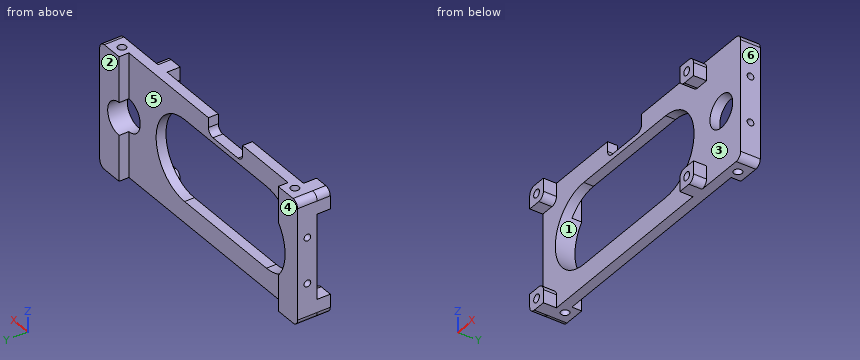
from build123d import *

# Parameters (mm, degrees)
BOSS_EXTRUDE1_DEPTH          = 38
FILLET3_R                    = 2
CUT_EXTRUDE1_DEPTH           = 98.349792201
CUT_EXTRUDE1_DEPTH_BACK      = 98.349792201
SKETCH3_W                    = 15
SKETCH3_H                    = 5
M3X0_5_TAPPED_HOLE3_D        = 2.5
M3X0_5_TAPPED_HOLE3_DEPTH    = 7.5
M3X0_5_TAPPED_HOLE3_TIP      = 0.751075774
M3X0_5_TAPPED_HOLE4_D        = 2.5
M3X0_5_TAPPED_HOLE4_DEPTH    = 7.5
M3X0_5_TAPPED_HOLE4_TIP      = 0.751075774
M2_5X0_45_TAPPED_HOLE1_D     = 2.05
M2_5X0_45_TAPPED_HOLE1_DEPTH = 6.35
M2_5X0_45_TAPPED_HOLE1_TIP   = 0.615882135
M2_5X0_45_TAPPED_HOLE2_D     = 2.05
M2_5X0_45_TAPPED_HOLE2_DEPTH = 6.35
M2_5X0_45_TAPPED_HOLE2_TIP   = 0.615882135
SKETCH14_R                   = 5
CUT_EXTRUDE2_DEPTH           = 98.488368751
SKETCH16_W                   = 6
SKETCH16_H                   = 6
BOSS_EXTRUDE2_DEPTH          = 4
FILLET4_R                    = 2
M3X0_5_TAPPED_HOLE5_D        = 2.5
M3X0_5_TAPPED_HOLE5_DEPTH    = 5.5
M3X0_5_TAPPED_HOLE5_TIP      = 0.751075774


with BuildPart() as part:
    # Sketch2 → Boss-Extrude1 (new body)
    with BuildSketch(Plane.XY.offset(11)):
        Polygon((-84.06534388, 85.95185693), (-75.56534388, 85.95185693), (-75.56534388, 82.95185693), (-5.56534388, 82.95185693), (-5.56534388, 85.95185693), (2.93465612, 85.95185693), (2.93465612, 79.95185693), (-84.06534388, 79.95185693), align=None)
    extrude(amount=BOSS_EXTRUDE1_DEPTH)

    # Fillet3
    fillet3_edges = [part.edges().sort_by_distance(p)[0] for p in [
        (2.93465612, 82.95185693, 49),
        (-84.06534388, 82.95185693, 11),
        (-84.06534388, 82.95185693, 49),
        (2.93465612, 82.95185693, 11),
    ]]
    fillet(fillet3_edges, radius=FILLET3_R)

    # Sketch3 → Cut-Extrude1 (cut, two sides: drawn at the far end of the back side and taken through both)
    with BuildSketch(Plane(origin=(0, 82.95185693, 0), x_dir=(1, 0, 0), z_dir=(0, 1, 0)).offset(-CUT_EXTRUDE1_DEPTH_BACK)):
        with BuildLine():
            Line((-66.06534388, -42.5), (-30.06534388, -42.5))
            ThreePointArc((-30.06534388, -42.5), (-17.56534388, -30), (-30.06534388, -17.5))
            Line((-30.06534388, -17.5), (-66.06534388, -17.5))
            ThreePointArc((-66.06534388, -17.5), (-78.56534388, -30), (-66.06534388, -42.5))
        make_face()
        with Locations((-48.06534388, -46.5)):
            Rectangle(SKETCH3_W, SKETCH3_H)
    extrude(amount=CUT_EXTRUDE1_DEPTH + CUT_EXTRUDE1_DEPTH_BACK, mode=Mode.SUBTRACT)

    # M3x0.5 Tapped Hole3
    with Locations(Plane.XY.offset(49)):
        with Locations((-78.56534388, 82.95185693), (-2.56534388, 82.95185693)):
            Hole(M3X0_5_TAPPED_HOLE3_D / 2, depth=M3X0_5_TAPPED_HOLE3_DEPTH)
            with Locations((0, 0, -(M3X0_5_TAPPED_HOLE3_DEPTH + M3X0_5_TAPPED_HOLE3_TIP / 2))):  # 118° drill point
                Cone(0, M3X0_5_TAPPED_HOLE3_D / 2, M3X0_5_TAPPED_HOLE3_TIP, mode=Mode.SUBTRACT)

    # M3x0.5 Tapped Hole4
    with Locations(Plane(origin=(0, 0, 11), x_dir=(-1, 0, 0), z_dir=(0, 0, -1))):
        with Locations((2.56534388, 82.95185693), (78.56534388, 82.95185693)):
            Hole(M3X0_5_TAPPED_HOLE4_D / 2, depth=M3X0_5_TAPPED_HOLE4_DEPTH)
            with Locations((0, 0, -(M3X0_5_TAPPED_HOLE4_DEPTH + M3X0_5_TAPPED_HOLE4_TIP / 2))):  # 118° drill point
                Cone(0, M3X0_5_TAPPED_HOLE4_D / 2, M3X0_5_TAPPED_HOLE4_TIP, mode=Mode.SUBTRACT)

    # M2.5x0.45 Tapped Hole1
    with Locations(Plane.ZY.offset(84.06534388)):
        with Locations((23, 82.95185693), (37, 82.95185693)):
            Hole(M2_5X0_45_TAPPED_HOLE1_D / 2, depth=M2_5X0_45_TAPPED_HOLE1_DEPTH)
            with Locations((0, 0, -(M2_5X0_45_TAPPED_HOLE1_DEPTH + M2_5X0_45_TAPPED_HOLE1_TIP / 2))):  # 118° drill point
                Cone(0, M2_5X0_45_TAPPED_HOLE1_D / 2, M2_5X0_45_TAPPED_HOLE1_TIP, mode=Mode.SUBTRACT)

    # M2.5x0.45 Tapped Hole2
    with Locations(Plane(origin=(2.93465612, 0, 0), x_dir=(0, 0, -1), z_dir=(1, 0, 0))):
        with Locations((-37, 82.95185693), (-23, 82.95185693)):
            Hole(M2_5X0_45_TAPPED_HOLE2_D / 2, depth=M2_5X0_45_TAPPED_HOLE2_DEPTH)
            with Locations((0, 0, -(M2_5X0_45_TAPPED_HOLE2_DEPTH + M2_5X0_45_TAPPED_HOLE2_TIP / 2))):  # 118° drill point
                Cone(0, M2_5X0_45_TAPPED_HOLE2_D / 2, M2_5X0_45_TAPPED_HOLE2_TIP, mode=Mode.SUBTRACT)

    # Sketch14 → Cut-Extrude2 (cut, through all)
    with BuildSketch(Plane(origin=(0, 85.95185693, 0), x_dir=(1, 0, 0), z_dir=(0, 1, 0))):
        with Locations(Location((-5.56534388, -30, 0), (0, 0, 270))):
            Circle(SKETCH14_R)
    extrude(amount=-CUT_EXTRUDE2_DEPTH, mode=Mode.SUBTRACT)

    # Sketch16 → Boss-Extrude2 (add)
    with BuildSketch(Plane.XZ.offset(-79.95185693)):
        with Locations((-81.06534388, 46)):
            Rectangle(SKETCH16_W, SKETCH16_H)
        with Locations((-81.06534388, 14)):
            Rectangle(SKETCH16_W, SKETCH16_H)
        with Locations((-15.06534388, 46)):
            Rectangle(SKETCH16_W, SKETCH16_H)
        with Locations((-15.06534388, 14)):
            Rectangle(SKETCH16_W, SKETCH16_H)
    extrude(amount=BOSS_EXTRUDE2_DEPTH)

    # Fillet4
    fillet4_edges = [part.edges().sort_by_distance(p)[0] for p in [
        (-12.06534388, 77.95185693, 11),
        (-84.06534388, 77.95185693, 11),
        (-84.06534388, 77.95185693, 49),
        (-78.06534388, 77.95185693, 43),
        (-78.06534388, 77.95185693, 17),
        (-18.06534388, 77.95185693, 17),
        (-18.06534388, 77.95185693, 43),
        (-12.06534388, 77.95185693, 49),
        (-40.56534388, 81.45185693, 44),
        (-55.56534388, 81.45185693, 44),
    ]]
    fillet(fillet4_edges, radius=FILLET4_R)

    # M3x0.5 Tapped Hole5
    with Locations(Plane.XZ.offset(-75.95185693)):
        with Locations((-81.06534388, 46), (-81.06534388, 14), (-15.06534388, 14), (-15.06534388, 46)):
            Hole(M3X0_5_TAPPED_HOLE5_D / 2, depth=M3X0_5_TAPPED_HOLE5_DEPTH)
            with Locations((0, 0, -(M3X0_5_TAPPED_HOLE5_DEPTH + M3X0_5_TAPPED_HOLE5_TIP / 2))):  # 118° drill point
                Cone(0, M3X0_5_TAPPED_HOLE5_D / 2, M3X0_5_TAPPED_HOLE5_TIP, mode=Mode.SUBTRACT)


solid = part.part
Geometry check sheet. Reference: the model listing, model coordinates, mm. Face numbers are marked on the shaded views. A direction names the side the tool comes from. Round coordinates to 2 decimals unless told otherwise and drop trailing zeros. Order: outer loops, then holes, each group sorted by start corner. A loop starts at its lowest first (then second) coordinate and runs counter-clockwise, first axis right, second up. Notation, with made-up numbers: (31.25, 41) -> (71.25, 41) arc R12 ccw to (71.25, 53) -> close; hole circle Ø5 at (-11, 74.5). An arc over 180 degrees is marked (long way). Use one line per item in the form item = value.
1. Cross-section at B-B, the plane y = 77. Enter the section's corners in (x, z), plus the area to 3 significant figures.
Working result:
outline = (-84.07, 13) arc R2 ccw to (-82.07, 11) -> (-78.07, 11) -> (-78.07, 15) arc R2 ccw to (-80.07, 17) -> (-84.07, 17) -> close; (-84.07, 43) -> (-80.07, 43) arc R2 ccw to (-78.07, 45) -> (-78.07, 49) -> (-82.07, 49) arc R2 ccw to (-84.07, 47) -> close; (-18.07, 11) -> (-14.07, 11) arc R2 ccw to (-12.07, 13) -> (-12.07, 17) -> (-16.07, 17) arc R2 ccw to (-18.07, 15) -> close; (-18.07, 45) arc R2 ccw to (-16.07, 43) -> (-12.07, 43) -> (-12.07, 47) arc R2 ccw to (-14.07, 49) -> (-18.07, 49) -> close; hole circle Ø2.5 at (-81.07, 14); hole circle Ø2.5 at (-81.07, 46); hole circle Ø2.5 at (-15.07, 14); hole circle Ø2.5 at (-15.07, 46)
area = 117 mm^2
2. Cross-section at C-C, the plane x = -63. Enter the section's corners in (y, z), plus the area to 3 significant figures.
Working result:
outline = (79.95, 11) -> (82.95, 11) -> (82.95, 17.5) -> (79.95, 17.5) -> close; (79.95, 42.5) -> (82.95, 42.5) -> (82.95, 49) -> (79.95, 49) -> close
area = 39.0 mm^2
3. Scan lines: line 1 along X through (y, z) = (82.75, 47); line 2 along X through (y, z) = (77.1, 46); line 3 along X through (y, z) = (85.75, 19.5). Record each from-to range of solid material in increasing order. Write a range as from..to.
Working result:
line_1 = -84.07..-79.8, -77.33..-55.57, -40.57..-3.8, -1.33..2.93
line_2 = -84.07..-82.32, -79.82..-78.07, -18.07..-16.32, -13.82..-12.07
line_3 = -84.07..-75.57, -5.57..2.93
4. Cross-section at D-D, the plane z = 32. Enter the section's corners in (x, y).
Working result:
outline = (-84.07, 79.95) -> (-78.4, 79.95) -> (-78.4, 85.95) -> (-84.07, 85.95) -> close; (-17.73, 79.95) -> (-10.15, 79.95) -> (-10.15, 82.95) -> (-17.73, 82.95) -> close; (-0.98, 79.95) -> (2.93, 79.95) -> (2.93, 85.95) -> (-0.98, 85.95) -> close
5. Go/stop test with flat-tipped pins: pin 1 (2 mm diameter, centred on x = -11, y = 78.5, fed in from -Z) (3 decimals); pin 2 (5 mm diameter, centred on x = -72.5, z = 16.5, fed in from +Y); pin 3 (3 mm diameter, centred on y = 78, z = 16, fed in from +X); pin 4 (2 mm diameter, centred on x = -2.57, y = 82.95, fed in from +Z). Record where each tip stops, or that it passes through.
Working result:
pin_1 = through
pin_2 = 82.95
pin_3 = -12.07
pin_4 = 41.35
6. Set-up check for the marked faces 1, 2 and 3: record each of +Z, -Z, +X, -X, +Y, -Y from which the full face is reachable in a straight line by a thin tool's end or side.
Working result:
face_1 = +Y, -Y
face_2 = +Z, -Z, +X, -X, +Y
face_3 = -Y
7. Cross-section at A-A, the plane y = 85. Enter the section's corners in (x, z), plus the area to 3 significant figures.
Working result:
outline = (-84.07, 13) arc R2 ccw to (-82.07, 11) -> (-75.57, 11) -> (-75.57, 21.88) arc R12.5 cw to (-75.57, 38.12) -> (-75.57, 49) -> (-82.07, 49) arc R2 ccw to (-84.07, 47) -> close; (-5.57, 11) -> (0.93, 11) arc R2 ccw to (2.93, 13) -> (2.93, 47) arc R2 ccw to (0.93, 49) -> (-5.57, 49) -> (-5.57, 35) arc R5 cw to (-5.57, 25) -> close
area = 570 mm^2
8. Mould release check, pull along X, two halves, no side actions. Record for the marked faces 4, 5 and 6: pulls with the +X half, pulls with the -X half, needs draft (parallel to the pull), parting line crosses it, or undercut.
Working result:
face_4 = needs draft
face_5 = undercut
face_6 = pulls with the +X half
